Here's how the part is built. I have some questions about the finished solid (model axes, mm). A direction names the side the tool comes from. Give positions to 0.01 mm unless a question says otherwise; leave off trailing zeros. Write each loop counter-clockwise with the first axis right and the second up, starting at its lowest first coordinate (ties: lowest second). Pieces come first, ordered by that corner, then holes. Notation, with made-up numbers: (32, -10.5) -> (76, -10.5) arc R10 ccw to (76, -5.5) -> close; hole circle Ø6 at (77.25, 24). An arc over 180 degrees is marked (long way). Return JSON: item names as keys, results as strings.
from build123d import *

# Parameters (mm, degrees)
F1_W        = 36.2
F1_H        = 68.8
F2_W        = 12.866667
F2_H        = 68.8
F4_DEPTH    = 12
F5_W        = 13.8
F5_H        = 13.8
F6_DEPTH    = 32
F7_T        = 3.6
F7_T3_DEPTH = 27.2
F7_T5_DEPTH = 21
F7_T7_DEPTH = 21


# Not quite as in the source:
# - a shell that OpenCascade refuses in one call is made with other operations: the cavity is built on its own and cut out


with BuildPart() as f3:
    # F1 (on offset) → F3 section 0
    with BuildSketch(Plane.XY.offset(36.125)):
        with Locations((0, -34.4)):
            Rectangle(F1_W, F1_H)
    # F2 (on Top) → F3 section 1
    with BuildSketch(Plane.XY):
        with Locations((-3.35e-05, -34.4)):
            Rectangle(F2_W, F2_H)
    loft()

    # F4 (cut): a face of the model
    f4_faces = [f3.faces().sort_by_distance(p)[0] for p in [
        (0, -34.4, 36.125),
    ]]
    extrude(f4_faces, amount=-F4_DEPTH, mode=Mode.SUBTRACT)

    # F5 (on offset) → F6 (cut)
    with BuildSketch(Plane.XY.offset(36.125)):
        with Locations((0, -34.4)):
            Rectangle(F5_W, F5_H)
    extrude(amount=-F6_DEPTH, mode=Mode.SUBTRACT)

    # F7: shell of thickness 3.6, made by hand


with BuildPart() as f7_core1:
    # F7_t2: copy of F3
    add(f3.part)

    # the walls: a layer under each face that stays
    f7_faces = [f7_core1.faces().sort_by_distance(p)[0] for p in [
        (-2.2314e-05, 0, 12.0625),
        (10.3289282007, -34.4, 12.0625),
        (-3.35e-05, -34.4, 0),
        (-10.3289728287, -34.4, 12.0625),
        (-2.2314e-05, -68.8, 12.0625),
        (0, -27.5, 14.125),
        (6.9, -34.4, 14.125),
        (0, -41.3, 14.125),
        (-6.9, -34.4, 14.125),
        (0, -34.4, 4.125),
    ]]
    thicken(f7_faces, amount=-F7_T, mode=Mode.SUBTRACT)

    # F7_s4 → F7_t3 (cut)
    with BuildSketch(Plane.XY.offset(0.525)):
        Polygon((-6.864, -27.536), (-6.9, -23.9), (-10.5, -23.9), (-10.5, -27.5), align=None)
        Polygon((6.864, -27.536), (6.9, -23.9), (10.5, -23.9), (10.5, -27.5), align=None)
        Polygon((6.864, -41.264), (10.5, -41.3), (10.5, -44.9), (6.9, -44.9), align=None)
        Polygon((-6.864, -41.264), (-6.9, -44.9), (-10.5, -44.9), (-10.5, -41.3), align=None)
    extrude(amount=F7_T3_DEPTH, mode=Mode.SUBTRACT)

    # F7_s6 → F7_t5 (cut)
    with BuildSketch(Plane.YZ.offset(-10.5)):
        Polygon((-27.536, 4.161), (-23.9, 4.125), (-23.9, 0.525), (-27.5, 0.525), align=None)
        Polygon((-41.264, 4.161), (-44.9, 4.125), (-44.9, 0.525), (-41.3, 0.525), align=None)
    extrude(amount=F7_T5_DEPTH, mode=Mode.SUBTRACT)

    # F7_s8 → F7_t7 (cut)
    with BuildSketch(Plane.XZ.offset(23.9)):
        Polygon((6.864, 4.161), (10.5, 4.125), (10.5, 0.525), (6.9, 0.525), align=None)
        Polygon((-6.864, 4.161), (-10.5, 4.125), (-10.5, 0.525), (-6.9, 0.525), align=None)
    extrude(amount=F7_T7_DEPTH, mode=Mode.SUBTRACT)


with BuildPart() as f3_1:
    add(f3.part)

    # what is left inside the walls is the cavity
    f7_cavity = [f7_core1.part.solids().sort_by_distance(p)[0] for p in [
        (8.197675, -13.75, 17.294397),
        (8.197675, -55.05, 17.294397),
    ]]
    add(f7_cavity, mode=Mode.SUBTRACT)


solid = f3_1.part
1. Suppose I cut it at A-A, the plane y = -29.5. List the corners of the cut face in (x, z) for me (3 decimals), and give its area (3 significant figures).
Taken from the geometry:
{"outline": "(-14.225, 24.125) -> (-6.433, 0) -> (6.433, 0) -> (14.225, 24.125) -> (6.9, 24.125) -> (6.9, 4.125) -> (-6.9, 4.125) -> (-6.9, 24.125) -> close", "area": "222 mm²"}
2. For pin 1 Ø7 at (y, z) = (-37.5, 18.5) entering from -X; pin 2 Ø4 at (x, y) = (-1, -60) entering from +Z; pin 3 Ø4 at (y, z) = (-31.5, 18) entering from -X, each with a flat end and sliding along its axis, tell me the tip position at first contact or that it passes through.
Taken from the geometry:
{"pin 1": "stops at x = -13.54", "pin 2": "stops at z = 3.6", "pin 3": "stops at x = -12.89"}
3. If we mould it in two halves opening along Y, with no side actions, what happens to faces 3 (the face through (0, -35, 0)), 4 (the face through (0, -44.9, 16))? For each: released by +Y, released by -Y, zero draft, split by the parting line, or undercut.
Taken from the geometry:
{"face 3": "zero draft", "face 4": "undercut"}
4. Suppose I cut it at C-C, the plane z = 10.5. Count the separate pieces of the cut face and the enclosed holes in it, and give its area (3 significant figures).
Taken from the geometry:
{"separate pieces": "1", "enclosed holes": "3", "area": "671 mm²"}
5. Suppose I cut it at B-B, the plane y = -11.5. List the corners of the cut face in (x, z) for me (1 decimal).
Taken from the geometry:
{"outline": "(-14.2, 24.1) -> (-6.4, 0) -> (6.4, 0) -> (14.2, 24.1) -> (10.4, 24.1) -> (3.8, 3.6) -> (-3.8, 3.6) -> (-10.4, 24.1) -> close"}
6. If I drill on line 1 (Y direction, x = -0.5, z = 9.5); line 2 (X direction, y = -18.5, z = 17.25); line 3 (X direction, y = -63.5, z = 17.75), over which ranges is the centre line in solid material (lowest first)? Write a range as [from, to].
Taken from the geometry:
{"line 1": "y = [-68.8, -65.2], [-44.9, -41.3], [-27.5, -23.9], [-3.6, 0]", "line 2": "x = [-12, -8.22], [8.22, 12]", "line 3": "x = [-12.17, -8.38], [8.38, 12.17]"}
7. Which directions (+Z, -Z, +X, -X, +Y, -Y) give clear straight access to the entire face, cutting with the end or side of a thin tool? Please do faces 1 (the face through (-7.1, -34, 24.125)), 2 (the face through (0, -14, 3.6)).
Taken from the geometry:
{"face 1": "+Z, +X, -X, +Y, -Y", "face 2": "+Z"}
